Source: CAD feature listing. Evaluate the final solid. Frame: model axes, mm. A direction names the side the tool comes from. Round coordinates to 2 decimals unless told otherwise and drop trailing zeros. Loops run counter-clockwise (first coordinate to the right, second up) from the corner with the lowest first, then second, coordinate; pieces in that order, holes last. Notation, with made-up numbers: M -32.75,-12 L -26.75,-12 A9 cw -26.75,3 Z; hole C -37.5,17.25 d8. An arc over 180 degrees is marked long. Write each question's results on one line, items separated by ' | '. Start each with the question number.
1. Set-up query: faces 4 (the cylindrical face through (-0.867, 3.905, -6.902)), 5 (the flat face through (-0.1, -2.4, 2)), 6 (the cylindrical face through (-1.08, -4.88, 10.49)). Return all of +Z, -Z, +X, -X, +Y, -Y with unobstructed straight access to the full face (end or side cutting, diameter ignored); none if empty.
2. Ray query, line 1 (Y direction, x = -0.25, z = 2.5); line 2 (Y direction, x = 0, z = -5.75); line 3 (X direction, y = 1.25, z = -3.25). Return the intervals inside material, ascending.
3. Draft query along Z for faces 1 (the flat face through (1, 2, -15)), 2 (the cylindrical face through (-1.19, -5.37, 5.94)), 3 (the cylindrical face through (0, 2, -6)). Return one class per face: released by +Z, released by -Z, zero draft, split by the parting line, or undercut.
4. Section A-A on y = 0. Output: boundary loops of the cut face in (x, z).
5. Section D-D on z = -12.5. Output: boundary loops of the cut face in (x, y), and give its area (3 significant figures).
6. Contact query for flat-ended pins moving along their axis: pin 1 Ø2 at (x, y) = (6, 3.5) entering from -Z; pin 2 Ø2 at (x, y) = (-2.5, 0) entering from +Z; pin 3 Ø3 at (y, z) = (-5, -4) entering from +X. Output: stop coordinate, or through.
7. Section C-C on z = 3. Output: boundary loops of the cut face in (x, y), and give its area (3 significant figures).
from build123d import *

# Parameters (mm, degrees)
F0_R     = 7.5
F1_DEPTH = 10
F2_R     = 4
F3_DEPTH = 15
F4_T     = -2
F5_R     = 7.5
F5_R_2   = 5
F6_DEPTH = 1
F8_SIZE  = 1
F9_SIZE  = 1


# Not quite as in the source:
# - a fillet or chamfer that OpenCascade refuses, or shapes differently, is made with other operations: its cross-section is extruded or revolved along the edge and cut away or added


with BuildPart() as f1:
    # F0 (on Top) → F1 (new body)
    with BuildSketch(Plane.XY):
        Circle(F0_R)
    extrude(amount=F1_DEPTH)

    # F2 (on face) → F3 (join)
    with BuildSketch(Plane(origin=(0, 0, 0), x_dir=(1, 0, 0), z_dir=(0, 0, -1))):
        Circle(F2_R)
    extrude(amount=F3_DEPTH)

    # F4
    f4_openings = [f1.faces().sort_by_distance(p)[0] for p in [
        (0, 0, 10),
        (0, 0, -15),
    ]]
    offset(amount=F4_T, openings=f4_openings, kind=Kind.INTERSECTION)

    # F5 (on face) → F6 (join)
    with BuildSketch(Plane.XY.offset(10)):
        Circle(F5_R)
        Circle(F5_R_2, mode=Mode.SUBTRACT)
    extrude(amount=F6_DEPTH)

    # F7: fillet of radius 3 on 1 edges, made by hand

    # F7_s1 → F7_t2 (revolve, cut)
    with BuildSketch(Plane.XZ):
        with BuildLine():
            ThreePointArc((7.5, 8.0419601084), (6.7912878475, 9.9784517816), (5, 11))
            Line((5, 11), (7.5, 11))
            Line((7.5, 11), (7.5, 8.0419601084))
        make_face()
    revolve(axis=Axis((0, 0, 11), (0, 0, 1)), mode=Mode.SUBTRACT)

    # F8
    f8_edges = [f1.edges().sort_by_distance(p)[0] for p in [
        (-7.5, 0, 0),
    ]]
    chamfer(f8_edges, length=F8_SIZE)

    # F9
    f9_edges = [f1.edges().sort_by_distance(p)[0] for p in [
        (-4, 0, -15),
    ]]
    chamfer(f9_edges, length=F9_SIZE)


solid = f1.part
Taken from the geometry:
1) face 4: -Z | face 5: none | face 6: +Z
2) line 1: -7.5 to -5.49, 5.49 to 7.5 | line 2: -4 to -2, 2 to 4 | line 3: -3.8 to -1.56, 1.56 to 3.8
3) face 1: released by -Z | face 2: undercut | face 3: zero draft
4) outline: M -7.5,1 L -6.5,0 L -4,0 L -4,-14 L -3,-15 L -2,-15 L -2,2 L -5.5,2 L -5.5,10 L -5,10 L -5,11 A3 ccw -7.5,8.04 Z; M 2,-15 L 3,-15 L 4,-14 L 4,0 L 6.5,0 L 7.5,1 L 7.5,8.04 A3 ccw 5,11 L 5,10 L 5.5,10 L 5.5,2 L 2,2 Z
5) outline: C 0,0 d8; hole C 0,0 d4 | area: 37.7 mm^2
6) pin 1: z = 0 | pin 2: z = 2 | pin 3: x = 1.94
7) outline: C 0,0 d15; hole C 0,0 d11 | area: 81.7 mm^2
